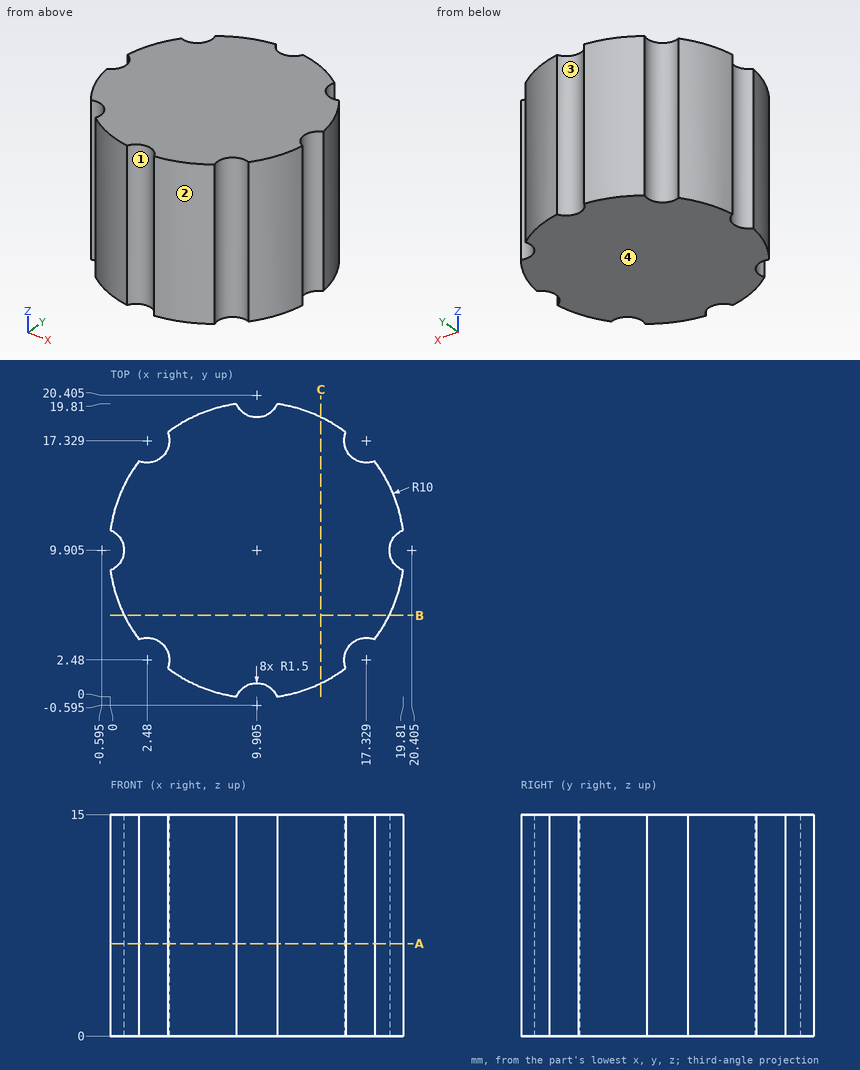
Source: three-view drawing plus pictorial views. Frame: mm from the lowest corner of the part. Coordinates: 2 decimals unless noted, no trailing zeros. Order: outer loops, then holes, each group sorted by start corner. A loop starts at its lowest first (then second) coordinate and runs counter-clockwise, first axis right, second up. Notation, with made-up numbers: M -33,18.5 L 2,18.5 A23 ccw 2,28.5 Z; hole C -21.75,-38.5 d7. An arc over 180 degrees is marked long. One line per question, with ' | ' between items.
Item 1: Draft query along X for the marked faces 1, 2, 3 and 4. Return one class per face: released by +X, released by -X, zero draft, split by the parting line, or undercut.
Geometry results:
face 1: undercut | face 2: released by +X | face 3: undercut | face 4: zero draft
Item 2: Section C-C (x = 14.25). Output: boundary loops of the cut face in (y, z).
Geometry results:
outline: M 0.9,0 L 18.91,0 L 18.91,15 L 0.9,15 Z
Item 3: Ray query, line 1 along X through (y, z) = (8.5, 12.25) (1 decimal); line 2 along Y through (x, z) = (15.5, 1) (1 decimal); line 3 along Y through (x, z) = (12.75, 9.25). Return the intervals inside material, ascending.
Geometry results:
line 1: x = 0 to 19.8 | line 2: y = 1.6 to 18.2 | line 3: y = 0.32 to 19.49
Item 4: Section A-A (z = 6.25). Output: boundary loops of the cut face in (x, y) (1 decimal), then the cut area to 3 significant figures.
Geometry results:
outline: M 0,8.5 A10 ccw 1.9,3.9 A1.5 cw 3.9,1.9 A10 ccw 8.5,0 A1.5 cw 11.3,0 A10 ccw 15.9,1.9 A1.5 cw 17.9,3.9 A10 ccw 19.8,8.5 A1.5 cw 19.8,11.3 A10 ccw 17.9,15.9 A1.5 cw 15.9,17.9 A10 ccw 11.3,19.8 A1.5 cw 8.5,19.8 A10 ccw 3.9,17.9 A1.5 cw 1.9,15.9 A10 ccw 0,11.3 A1.5 cw Z | area: 298 mm^2
Item 5: Section B-B (y = 5.5). Output: boundary loops of the cut face in (x, z).
Geometry results:
outline: M 0.93,0 L 18.88,0 L 18.88,15 L 0.93,15 Z
Item 6: Pin query (flat end, axial travel): pin 1 (5 mm diameter, centred on x = 17.5, z = 1.5, fed in from -Y); pin 2 (2 mm diameter, centred on y = 7.5, z = 13.5, fed in from -X); pin 3 (2 mm diameter, centred on y = 14, z = 7, fed in from -X) (1 decimal). Return the tip coordinate at first contact, or that it passes through.
Geometry results:
pin 1: stops at y = 1.3 | pin 2: stops at x = 0 | pin 3: stops at x = 0.4
